The model under review builds one solid part; all positions refer to its coordinate system, in mm. A direction names the side the tool comes from. Round coordinates to 2 decimals unless told otherwise and drop trailing zeros. Write each loop counter-clockwise with the first axis right and the second up, starting at its lowest first coordinate (ties: lowest second). Pieces come first, ordered by that corner, then holes. Notation, with made-up numbers: (39, 22.25) -> (97, 22.25) arc R31 cw to (97, 61.25) -> close; hole circle Ø4 at (56.5, 4). An arc over 180 degrees is marked (long way). Answer in a Markdown table with one row per item. Add a question column.
```python
from build123d import *

# Parameters (mm, degrees)
SKETCH1_R           = 9.5
BOSS_EXTRUDE1_DEPTH = 15.5
BOSS_EXTRUDE2_REACH = 167.695
SKETCH2_R           = 31
CUT_EXTRUDE1_REACH  = 167.695
SKETCH3_R           = 17.5


with BuildPart() as part:
    # Sketch1 → Boss-Extrude1 (new body)
    with BuildSketch(Plane(origin=(0, 0, 0), x_dir=(1, 0, 0), z_dir=(0, 1, 0))):
        with BuildLine():
            Line((-85, -50), (-19.5, -50))
            Line((-19.5, -50), (-19.5, -72))
            ThreePointArc((-19.5, -72), (0, -91.5), (19.5, -72))
            Line((19.5, -72), (19.5, -50))
            Line((19.5, -50), (85, -50))
            ThreePointArc((85, -50), (95.606601718, -45.606601718), (100, -35))
            Line((100, -35), (100, 35))
            ThreePointArc((100, 35), (95.606601718, 45.606601718), (85, 50))
            Line((85, 50), (19.5, 50))
            Line((19.5, 50), (19.5, 72))
            ThreePointArc((19.5, 72), (0, 91.5), (-19.5, 72))
            Line((-19.5, 72), (-19.5, 50))
            Line((-19.5, 50), (-85, 50))
            ThreePointArc((-85, 50), (-95.606601718, 45.606601718), (-100, 35))
            Line((-100, 35), (-100, -35))
            ThreePointArc((-100, -35), (-95.606601718, -45.606601718), (-85, -50))
        make_face()
        with Locations(Location((0, -72, 0), (0, 0, 270))):
            Circle(SKETCH1_R, mode=Mode.SUBTRACT)
        with Locations(Location((0, 72, 0), (0, 0, 90))):
            Circle(SKETCH1_R, mode=Mode.SUBTRACT)
    extrude(amount=-BOSS_EXTRUDE1_DEPTH)

    # Boss-Extrude2: up to this plane
    boss_extrude2_end = Plane(origin=(0, 0, 72), z_dir=(0, 1, 0))
    # Sketch2 → Boss-Extrude2 (add, up to the surface)
    with BuildSketch(Plane(origin=(25, 43.301270189, 0), x_dir=(0, 0, -1), z_dir=(0.500000000000001, 0.866025403784438, 0)), mode=Mode.PRIVATE) as boss_extrude2_sk1:
        with Locations(Location((0, 13.397459622, 0), (0, 0, 90))):
            Circle(SKETCH2_R)
    boss_extrude2_tool1 = split(extrude(boss_extrude2_sk1.sketch, amount=-BOSS_EXTRUDE2_REACH, mode=Mode.PRIVATE), bisect_by=boss_extrude2_end, keep=Keep.BOTH, mode=Mode.PRIVATE)
    add(boss_extrude2_tool1.solids().sort_by_distance((13.39746, 50, 0))[0])

    # Cut-Extrude1: up to this plane
    cut_extrude1_end = Plane(origin=(0, -15.5, 72), z_dir=(0, 1, 0))
    # Sketch3 → Cut-Extrude1 (cut, up to the surface)
    with BuildSketch(Plane(origin=(25, 43.301270189, 0), x_dir=(0.8660254037844382, -0.500000000000001, 0), z_dir=(0.500000000000001, 0.8660254037844382, 0)), mode=Mode.PRIVATE) as cut_extrude1_sk1:
        with Locations(Location((-13.397459622, 0, 0), (0, 0, 180))):
            Circle(SKETCH3_R)
    cut_extrude1_tool1 = split(extrude(cut_extrude1_sk1.sketch, amount=-CUT_EXTRUDE1_REACH, mode=Mode.PRIVATE), bisect_by=cut_extrude1_end, keep=Keep.BOTH, mode=Mode.PRIVATE)
    add(cut_extrude1_tool1.solids().sort_by_distance((13.39746, 50, 0))[0], mode=Mode.SUBTRACT)


solid = part.part
```
1. Add section A-A on z = -13.5. Write out the cut boundary in (x, y).
2. For L1, parallel to X at y = -5, z = 72; L2, parallel to Z at x = -3.5, y = 18; L3, parallel to Y at x = 42.5, z = 20.5, list the stretches that pass through material, from the lowest coordinate up.
3. Add section B-B on x = -64. Write out the cut boundary in (y, z).
4. Add section C-C on z = -69.5. Write out the cut boundary in (x, y).
5. Mouldability with a two-part tool opening along Y and no side actions: class faces 1 (the cylindrical face through (-26.65, 39.77, 9.31)), 2 (the flat face through (1.841, 56.672, -13.344)), 3 (the flat face through (52, -8, 50)), 4 (the flat face through (-1, -15.5, -1)) as pulls with the +Y half, pulls with the -Y half, needs draft (parallel to the pull), parting line crosses it, or undercut.
6. Insertion check: pin 1 Ø17 at (x, y) = (-52, -10) entering from -Z; pin 2 Ø4.5 at (x, y) = (-51, -6) entering from +Z; pin 3 Ø3 at (x, z) = (18, -65) entering from +Y. Each pin has a flat end and moves straight along its axis. Give the tip position at first contact, or say it passes through.
7. Tool access review of faces 5 (the flat face through (53, -8, -50)), 6 (the flat face through (-52, -8, -50)), 7 (the flat face through (-53, -8, 50)): name each direction out of +Z, -Z, +X, -X, +Y, -Y from which nothing blocks a thin tool from reaching the whole face with its end or side.
8. Add section D-D on y = -4. State how many separate pieces and enclosed holes the cut face has, plus the area to 3 significant figures.
Filled in:
| question | item | result |
|---|---|---|
| 1 | outline | (-100, -15.5) -> (-37.28, -15.5) -> (3.75, 55.57) -> (-10.77, 63.95) -> (-47.69, 0) -> (-100, 0) -> close; (-11.56, -15.5) -> (100, -15.5) -> (100, 0) -> (16.75, 0) -> (37.56, 36.05) -> (23.04, 44.43) -> close |
| 2 | L1 | -19.5 to -9.5, 9.5 to 19.5 |
| 2 | L2 | -30.97 to -17.45, 17.45 to 30.97 |
| 2 | L3 | -15.5 to 0 |
| 3 | outline | (-15.5, -50) -> (0, -50) -> (0, 50) -> (-15.5, 50) -> close |
| 4 | outline | (-19.5, -15.5) -> (-9.17, -15.5) -> (-9.17, 0) -> (-19.5, 0) -> close; (9.17, -15.5) -> (19.5, -15.5) -> (19.5, 0) -> (9.17, 0) -> close |
| 5 | face 1 | undercut |
| 5 | face 2 | pulls with the +Y half |
| 5 | face 3 | needs draft |
| 5 | face 4 | pulls with the -Y half |
| 6 | pin 1 | z = -50 |
| 6 | pin 2 | z = 50 |
| 6 | pin 3 | y = 0 |
| 7 | face 5 | -Z, +X, +Y, -Y |
| 7 | face 6 | -Z, -X, +Y, -Y |
| 7 | face 7 | +Z, -X, +Y, -Y |
| 8 | separate pieces | 1 |
| 8 | enclosed holes | 3 |
| 8 | area | 21,000 mm² |
